Job drawing, mm, ordinate dimensions from the low corner. One solid piece. Give positions to 0.01 mm unless a question says otherwise; leave off trailing zeros. Order: outer loops, then holes, each group sorted by start corner. A loop starts at its lowest first (then second) coordinate and runs counter-clockwise, first axis right, second up. Notation, with made-up numbers: M 30.25,-15.5 L 54.25,-15.5 A22 ccw 54.25,15.5 Z; hole C 39.25,-31 d8. An arc over 180 degrees is marked long. Put each result on its own line as item: value. Start each with the question number.
1) Cut at A-A (x = 5.5). Write the cut outline in (y, z), and give its area (3 significant figures).
2) Drill centre lines: line 1 (X direction, y = 5, z = 2.4); line 2 (Y direction, x = 14.5, z = 2.4); line 3 (X direction, y = 6, z = 3.8). Where is each one in solid material? Low to high. Write a range as [from, to].
3) Two-plate mould, pull along X, no slides. Class the marked faces 1, 2, 3 and 4: released by +X, released by -X, zero draft, split by the parting line, or undercut.
4) Cut at C-C (z = 1.6). Write the cut outline in (x, y), and give its area (3 significant figures).
5) Pin check, flat tip, straight feed: pin 1 (1.5 mm diameter, centred on x = 9, z = 1, fed in from -Y). Stop position of the tip, or through.
6) Cut at B-B (y = 5). Write the cut outline in (x, z), and give its area (3 significant figures).
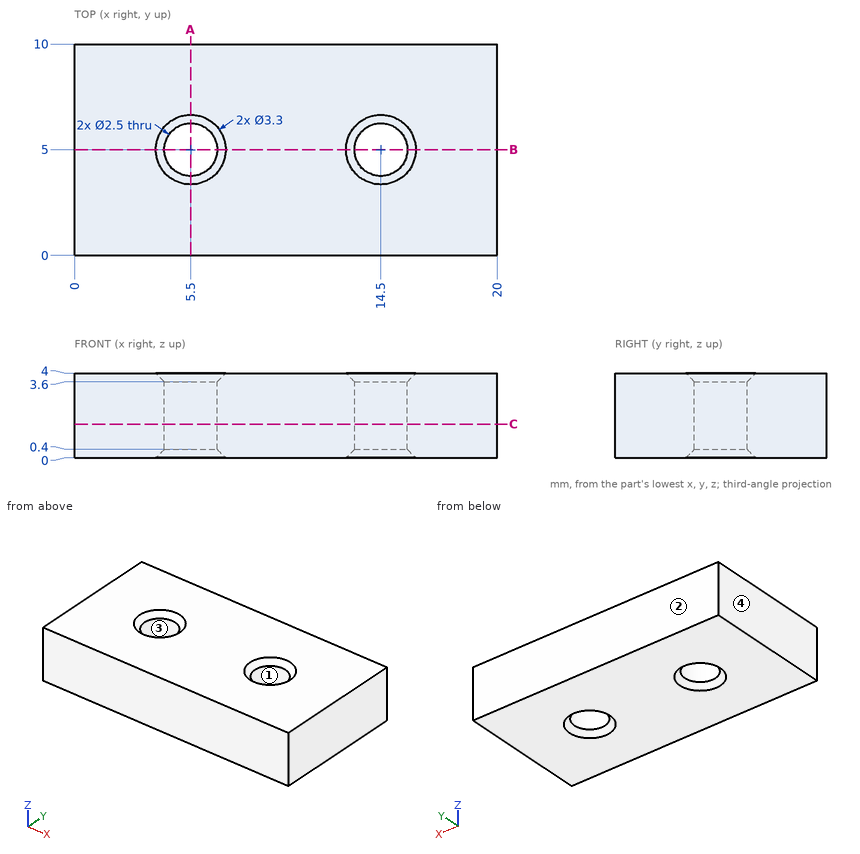
Solution:
1. outline: M 0,0 L 3.35,0 L 3.75,0.4 L 3.75,3.6 L 3.35,4 L 0,4 Z; M 6.25,0.4 L 6.65,0 L 10,0 L 10,4 L 6.65,4 L 6.25,3.6 Z
1. area: 29.7 mm²
2. line 1: [0, 4.25], [6.75, 13.25], [15.75, 20]
2. line 2: [0, 3.75], [6.25, 10]
2. line 3: [0, 4.45], [6.55, 13.45], [15.55, 20]
3. face 1: undercut
3. face 2: zero draft
3. face 3: undercut
3. face 4: released by -X
4. outline: M 0,0 L 20,0 L 20,10 L 0,10 Z; hole C 5.5,5 d2.5; hole C 14.5,5 d2.5
4. area: 190 mm²
5. pin 1: y = 0
6. outline: M 0,0 L 3.85,0 L 4.25,0.4 L 4.25,3.6 L 3.85,4 L 0,4 Z; M 6.75,0.4 L 7.15,0 L 12.85,0 L 13.25,0.4 L 13.25,3.6 L 12.85,4 L 7.15,4 L 6.75,3.6 Z; M 15.75,0.4 L 16.15,0 L 20,0 L 20,4 L 16.15,4 L 15.75,3.6 Z
6. area: 59.4 mm²
